Could you check a few things on this model? Use its own coordinates, in mm. Give positions to 0.01 mm unless a question says otherwise; leave off trailing zeros. Order: outer loops, then holes, each group sorted by start corner. A loop starts at its lowest first (then second) coordinate and runs counter-clockwise, first axis right, second up. Notation, with made-up numbers: M 81.5,7 L 120.5,7 A20 cw 120.5,18 Z; hole C 25.25,26 d9. An arc over 180 degrees is marked long. Answer in a Markdown table with one row per item. Add a question column.
```python
from build123d import *

# Parameters (mm, degrees)
BOX006_W        = 48
BOX006_H        = 35
BOX006_DEPTH    = 10
SKETCH007_R     = 3.8
POCKET001_DEPTH = 10
FILLET007_R     = 1.5


with BuildPart() as part:
    # Box006 → Box006 (new body)
    with BuildSketch(Plane(origin=(-24, -22, -15), x_dir=(1, 0, 0), z_dir=(0, 0, 1))):
        with Locations((24, 17.5)):
            Rectangle(BOX006_W, BOX006_H)
    extrude(amount=BOX006_DEPTH)

    # Sketch007 → Pocket001 (cut)
    with BuildSketch(Plane(origin=(-24, -22, -15), x_dir=(1, 0, 0), z_dir=(0, 0, -1))):
        with Locations((24, -17.5)):
            Circle(SKETCH007_R)
    extrude(amount=-POCKET001_DEPTH, mode=Mode.SUBTRACT)

    # Fillet007
    fillet007_edges = [part.edges().sort_by_distance(p)[0] for p in [
        (-24, -22, -10),
        (-24, 13, -10),
        (24, -22, -10),
        (0, 13, -15),
        (-24, -4.5, -15),
        (-3.8, -4.5, -5),
        (0, -22, -15),
        (24, 13, -10),
    ]]
    fillet(fillet007_edges, radius=FILLET007_R)


solid = part.part
```
1. If I drill on line 1 along X through (y, z) = (-4.5, -11.75); line 2 along Y through (x, z) = (0, -9.75); line 3 along X through (y, z) = (-6.5, -6.5), over which ranges is the centre line in solid material (lowest first)? Write a range as [from, to].
2. Suppose I cut it at A-A on y = -4.5. List the corners of the cut face in (x, z) for me.
3. Will this pin go through, and if not, where does the flat tip stop? P1, Ø4.5, axis at x = 0, y = -4.5, coming from the +Z side.
4. Thinking about a two-plate mould opening in Y: for faces 1 (the flat face through (-5, -4, -15)), 2 (the cylindrical face through (-2.8, -7.07, -10.81)), 3 (the cylindrical face through (-23.57, -21.55, -9.19)), which applies, pulls with the +Y half, pulls with the -Y half, needs draft (parallel to the pull), parting line crosses it, or undercut?
5. Suppose I cut it at D-D on z = -6. List the corners of the cut face in (x, y) for me.
6. Suppose I cut it at B-B on x = 0. List the corners of the cut face in (y, z) for me.
7. Suppose I cut it at C-C on z = -12. List the corners of the cut face in (x, y) for me.
Findings below:
| question | item | result |
|---|---|---|
| 1 | line 1 | [-24, -3.8], [3.8, 24] |
| 1 | line 2 | [-22, -8.3], [-0.7, 13] |
| 1 | line 3 | [-24, -3.23], [3.23, 24] |
| 2 | outline | M -24,-13.5 A1.5 ccw -22.5,-15 L -3.8,-15 L -3.8,-6.5 A1.5 ccw -5.3,-5 L -24,-5 Z; M 3.8,-15 L 24,-15 L 24,-5 L 5.3,-5 A1.5 ccw 3.8,-6.5 Z |
| 3 | P1 | through |
| 4 | face 1 | needs draft |
| 4 | face 2 | undercut |
| 4 | face 3 | pulls with the -Y half |
| 5 | outline | M -24,-20.5 A1.5 ccw -22.5,-22 L 22.5,-22 A1.5 ccw 24,-20.5 L 24,11.5 A1.5 ccw 22.5,13 L -22.5,13 A1.5 ccw -24,11.5 Z; hole C 0,-4.5 d7.77 |
| 6 | outline | M -22,-13.5 A1.5 ccw -20.5,-15 L -8.3,-15 L -8.3,-6.5 A1.5 ccw -9.8,-5 L -22,-5 Z; M -0.7,-15 L 11.5,-15 A1.5 ccw 13,-13.5 L 13,-5 L 0.8,-5 A1.5 ccw -0.7,-6.5 Z |
| 7 | outline | M -24,-20.5 A1.5 ccw -22.5,-22 L 22.5,-22 A1.5 ccw 24,-20.5 L 24,11.5 A1.5 ccw 22.5,13 L -22.5,13 A1.5 ccw -24,11.5 Z; hole C 0,-4.5 d7.6 |
